Drawing for the job (mm, zero at the part's lowest x, y, z). Give positions to 0.01 mm unless a question says otherwise; leave off trailing zeros. Order: outer loops, then holes, each group sorted by start corner. A loop starts at its lowest first (then second) coordinate and runs counter-clockwise, first axis right, second up. Notation, with made-up numbers: (56, -27.5) - (85, -27.5) arc R22 cw to (85, 2.5) - close; hole circle Ø2 at (68.25, 78). An arc over 180 degrees is marked (long way). Use a Markdown table: item, result.
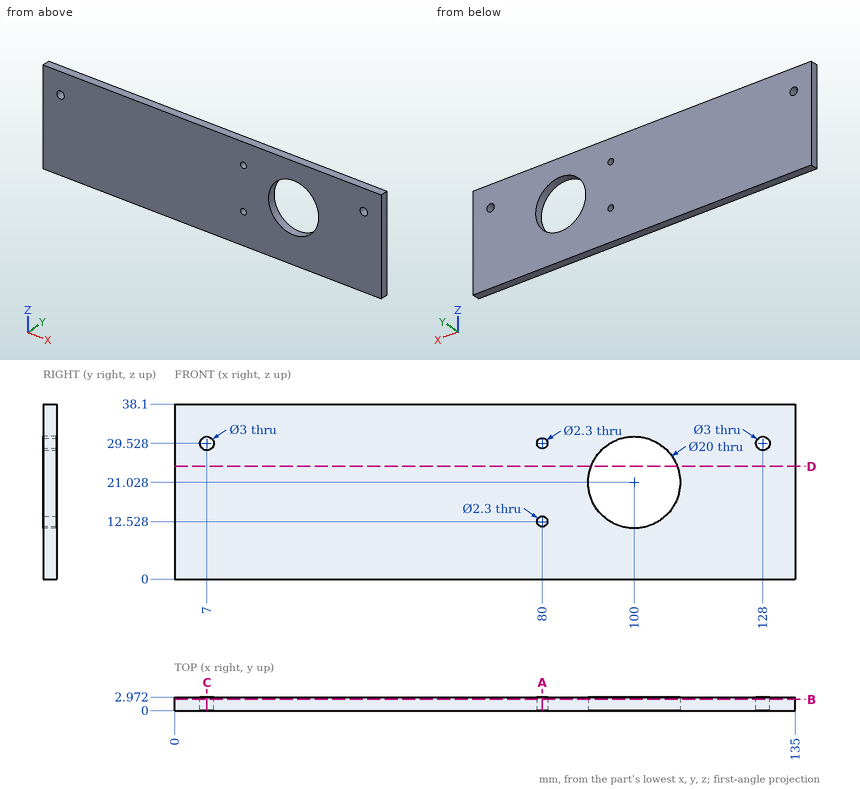
1) Wall check: line 1 (Z direction, x = 128, y = 1.65); line 2 (Z direction, x = 6, y = 1.5); line 3 (X direction, y = 0.5, z = 12). Give the ranges that are in metal, low to high. Write a range as from..to.
Computed:
| item | result |
|---|---|
| line 1 | z = 0..28.03, 31.03..38.1 |
| line 2 | z = 0..28.41, 30.65..38.1 |
| line 3 | x = 0..78.98, 81.02..95.7, 104.3..135 |
2) Slice it at D-D (z = 24.5). Write the cut outline in (x, y).
Computed:
| item | result |
|---|---|
| outline | (0, 0) - (90.62, 0) - (90.62, 2.97) - (0, 2.97) - close; (109.38, 0) - (135, 0) - (135, 2.97) - (109.38, 2.97) - close |
3) Slice it at B-B (y = 2.45). Write the cut outline in (x, z).
Computed:
| item | result |
|---|---|
| outline | (0, 0) - (135, 0) - (135, 38.1) - (0, 38.1) - close; hole circle Ø3 at (7, 29.53); hole circle Ø2.3 at (80, 12.53); hole circle Ø2.3 at (80, 29.53); hole circle Ø20 at (100, 21.03); hole circle Ø3 at (128, 29.53) |
4) Pin check, flat tip, straight feed: P1, Ø1, axis at x = 95, z = 28.5, coming from the -Y side. Stop position of the tip, or through.
Computed:
| item | result |
|---|---|
| P1 | passes through |
5) Slice it at A-A (x = 80). Write the cut outline in (y, z).
Computed:
| item | result |
|---|---|
| outline | (0, 0) - (2.97, 0) - (2.97, 11.38) - (0, 11.38) - close; (0, 13.68) - (2.97, 13.68) - (2.97, 28.38) - (0, 28.38) - close; (0, 30.68) - (2.97, 30.68) - (2.97, 38.1) - (0, 38.1) - close |
6) Slice it at C-C (x = 7). Write the cut outline in (y, z).
Computed:
| item | result |
|---|---|
| outline | (0, 0) - (2.97, 0) - (2.97, 28.03) - (0, 28.03) - close; (0, 31.03) - (2.97, 31.03) - (2.97, 38.1) - (0, 38.1) - close |
